Autodesk Inventor part; units mm, degrees
ref_plane "YZ Plane" through (0, 0, 0) normal (1, 0, 0) x (0, 1, 0)
ref_plane "XZ Plane" through (0, 0, 0) normal (0, 1, 0) x (-1, 0, 0)
ref_plane "XY Plane" through (0, 0, 0) normal (0, 0, 1) x (1, 0, 0)
sketch "Sketch1" plane through (0, 0, 0) normal (0, 0, 1) x (1, 0, 0)
  circle A0 centre (0, 0) radius 12.7
  circle A1 centre (0, 0) radius 50.8
  line L0 (50.8, 0) -> (50.8, -225.3234)
  line L1 (50.8, -225.3234) -> (-50.8, -225.3234)
  line L2 (-50.8, -225.3234) -> (-50.8, 0)
  line L3 (-50.8, 0) -> (-12.7, 0)
  line L4 (12.7, 0) -> (50.8, 0)
  dimension "d1" = 101.6
  dimension "d0" = 25.4
  dimension "d2" = 225.3234
extrude "Extrusion1" add sketch "Sketch1" along normal blind 12.7 contours L4 A1 L3 A0 | A0 L3 A1 L4 | L0 L1 L2 A1
sketch "Sketch2" plane through (0, 0, 12.7) normal (0, 0, 1) x (1, 0, 0)
  circle A0 centre (0, 0) radius 12.7
  arc A1 (50.8, 0) -> (-50.8, 0) centre (0, 0) ccw
  line L0 (-50.8, 0) -> (-50.8, -225.3234)
  line L1 (-50.8, -225.3234) -> (50.8, -225.3234)
  line L2 (50.8, -225.3234) -> (50.8, 0)
  circle A2 centre (176.5046, -179.1208) radius 32.385
  circle A3 centre (253.9746, -179.1208) radius 32.385
  line L3 (144.1196, -225.3234) -> (144.1196, -179.1208)
  line L4 (286.3596, -225.3234) -> (286.3596, -179.1208)
  line L5 (176.5046, -146.7358) -> (253.9746, -146.7358)
  line L6 (50.8, -225.3234) -> (144.1196, -225.3234)
  line L7 (286.3596, -225.3234) -> (508, -225.3234)
  line L8 (-50.8, -225.3234) -> (-238.2266, -225.3234)
  line L9 (-263.6266, -225.3234) -> (-263.6266, -150.876)
  line L10 (-263.6266, -150.876) -> (-212.8266, -150.876)
  line L11 (-212.8266, -150.876) -> (-212.8266, 50.8)
  line L12 (-212.8266, 50.8) -> (508, 50.8)
  line L13 (508, 50.8) -> (508, -225.3234)
  line L14 (-238.2266, -229.108) -> (-238.2266, -225.3234)
  line L15 (-238.2266, -229.108) -> (-263.6266, -229.108)
  line L16 (-263.6266, -229.108) -> (-263.6266, -225.3234)
  dimension "d5" = 176.5046
  dimension "d6" = 179.1208
  dimension "d7" = 64.77
  dimension "d8" = 64.77
  dimension "d9" = 77.47
  dimension "d11" = 212.8266
  dimension "d13" = 50.8
  dimension "d16" = 150.876
  dimension "d17" = 508
  dimension "d18" = 229.108
extrude "Extrusion2" add sketch "Sketch2" against normal blind 12.7 contours A1 L12 L13 L7 L4 A3 L5 A2 L3 L6 L2 | A1 L0 L8 L14 L15 L16 L9 L10 L11 L12
sketch "Sketch3" plane through (0, 0, 12.7) normal (0, 0, 1) x (1, 0, 0)
  circle A0 centre (0, 0) radius 12.7
  circle A1 centre (225.0958, -205.5114) radius 12.7
  dimension "d19" = 25.4
  dimension "d20" = 304.8
  dimension "d21" = 205.5114
sketch "Sketch4" plane through (0, 0, 12.7) normal (0, 0, 1) x (1, 0, 0)
  line L0 (144.1196, -225.3234) -> (106.0196, -225.3234)
  line L1 (106.0196, -225.3234) -> (106.0196, -136.4234)
  line L2 (106.0196, -136.4234) -> (144.1196, -136.4234)
  line L3 (144.1196, -136.4234) -> (144.1196, -225.3234)
  line L4 (286.3596, -225.3234) -> (324.4596, -225.3234)
  line L5 (324.4596, -225.3234) -> (324.4596, -136.4234)
  line L6 (324.4596, -136.4234) -> (286.3596, -136.4234)
  line L7 (286.3596, -136.4234) -> (286.3596, -225.3234)
  dimension "d22" = 38.1
  dimension "d23" = 88.9
  dimension "d24" = 38.1
  dimension "d25" = 88.9
extrude "Extrusion3" add sketch "Sketch4" along normal blind 25.4
sketch "Sketch5" plane through (0, 0, 38.1) normal (0, 0, 1) x (1, 0, 0)
  line L0 (106.0196, -136.4234) -> (324.4596, -136.4234)
  line L1 (324.4596, -136.4234) -> (324.4596, -225.3234)
  line L2 (324.4596, -225.3234) -> (106.0196, -225.3234)
  line L3 (106.0196, -225.3234) -> (106.0196, -136.4234)
  point P0 (0, 0)
  dimension "d28" = 218.44
extrude "Extrusion4" add sketch "Sketch5" along normal blind 12.7
extrude "Extrusion5" cut sketch "Sketch3" along normal blind 76.2 contours A1
sketch "Sketch6" plane through (0, 0, 12.7) normal (0, 0, 1) x (1, 0, 0)
  line L0 (324.4596, -136.4234) -> (324.4596, -225.3234)
  line L1 (324.4596, -225.3234) -> (508, -225.3234)
  line L2 (508, -225.3234) -> (508, 50.8)
  line L3 (324.4596, -136.4234) -> (508, -22.1234)
  dimension "d33" = 203.2
extrude "Extrusion6" cut sketch "Sketch6" against normal blind 25.4
sketch "Sketch7" plane through (0, 0, 50.8) normal (0, 0, 1) x (1, 0, 0)
  line L0 (106.0196, -136.4234) -> (106.0196, -225.3234)
  line L1 (324.4596, -225.3234) -> (324.4596, -136.4234)
  line L2 (324.4596, -136.4234) -> (106.0196, -136.4234)
  arc A0 (324.4596, -225.3234) -> (235.5596, -136.4234) centre (235.5596, -225.3234) ccw
  line L3 (324.4596, -225.3234) -> (235.5596, -136.4234) construction
  line L4 (324.4596, -225.3234) -> (450.1832, -225.3234) construction
  arc A1 (194.9196, -136.4234) -> (106.0196, -225.3234) centre (194.9196, -225.3234) ccw
  line L5 (106.0196, -225.3234) -> (194.9196, -136.4234) construction
  line L6 (106.0196, -225.3234) -> (231.7432, -225.3234) construction
  point P0 (0, 0)
  dimension "d36" = 135
  dimension "d37" = 45
extrude "Extrusion7" cut sketch "Sketch7" against normal blind 38.1
fillet "Fillet1" radius 12.7 3 edges at (215.2396, -136.4234, 50.8) (298.4214, -162.4616, 50.8) (132.0578, -162.4616, 50.8)
sketch "Sketch8" plane through (0, 0, 0) normal (0, 0, -1) x (-1, 0, 0)
  line L0 (-508, 50.8) -> (-508, -22.1234)
  circle A0 centre (0, 0) radius 12.7
  line L1 (0, 0) -> (-271.2669, 0)
  circle A1 centre (-271.2669, 0) radius 35.56
  dimension "d41" = 71.12
extrude "Extrusion8" cut sketch "Sketch8" against normal blind 25.4 contours A1
sketch "Sketch9" plane through (0, 0, 0) normal (0, 0, -1) x (-1, 0, 0)
  circle A0 centre (-271.2669, 0) radius 35.56
  line L0 (-324.4596, -136.4234) -> (-324.4596, -225.3234)
  line L1 (-324.4596, -225.3234) -> (-286.3596, -225.3234)
  line L2 (-286.3596, -225.3234) -> (-286.3596, -179.1208)
  arc A1 (-253.9746, -146.7358) -> (-286.3596, -179.1208) centre (-253.9746, -179.1208) ccw
  line L3 (-253.9746, -146.7358) -> (-176.5046, -146.7358)
  arc A2 (-144.1196, -179.1208) -> (-176.5046, -146.7358) centre (-176.5046, -179.1208) ccw
  line L4 (-144.1196, -179.1208) -> (-144.1196, -225.3234)
  line L5 (-144.1196, -225.3234) -> (238.2266, -225.3234)
  line L6 (238.2266, -225.3234) -> (238.2266, -229.108)
  line L7 (238.2266, -229.108) -> (263.6266, -229.108)
  line L8 (263.6266, -229.108) -> (263.6266, -150.876)
  line L9 (263.6266, -150.876) -> (212.8266, -150.876)
  line L10 (212.8266, -150.876) -> (212.8266, 50.8)
  line L11 (212.8266, 50.8) -> (-508, 50.8)
  line L12 (-508, 50.8) -> (-508, -22.1234)
  line L13 (-508, -22.1234) -> (-324.4596, -136.4234)
  circle A3 centre (0, 0) radius 12.7
properties part number "Shooter_TopMotorSupport"
Input: part model. Units: mm. Frame: model coordinates. A direction names the side the tool comes from. Give positions to 0.01 mm unless a question says otherwise; leave off trailing zeros. Order: outer loops, then holes, each group sorted by start corner. A loop starts at its lowest first (then second) coordinate and runs counter-clockwise, first axis right, second up.
1. Section C-C on z = 22. Return the cut outline in (x, y).
Derived:
outline: (106.02, -225.32) - (144.12, -225.32) - (144.12, -152.37) arc R88.9 ccw to start; (286.36, -225.32) - (324.46, -225.32) arc R88.9 ccw to (286.36, -152.37) - close
2. Section A-A on y = 0. Return the cut outline in (x, z), and give its area (3 significant figures).
Derived:
outline: (-212.83, 0) - (-12.7, 0) - (-12.7, 12.7) - (-212.83, 12.7) - close; (12.7, 0) - (235.71, 0) - (235.71, 12.7) - (12.7, 12.7) - close; (306.83, 0) - (508, 0) - (508, 12.7) - (306.83, 12.7) - close
area: 7,930 mm2
3. Pin query (flat end, axial travel): pin 1 (4 mm diameter, centred on x = 141, z = 26.5, fed in from +Y); pin 2 (1 mm diameter, centred on x = 342, z = 7.5, fed in from -Y); pin 3 (5 mm diameter, centred on x = 313, z = 35.5, fed in from -Y). Return the tip coordinate at first contact, or that it passes through.
Derived:
pin 1: stops at y = -153.16
pin 2: stops at y = -125.81
pin 3: stops at y = -225.32
4. Material intervals for L1, parallel to X at y = -177, z = 10; L2, parallel to Y at x = 308, z = 2; L3, parallel to Y at x = 233, z = 8, sorted ascending.
Derived:
L1: x = -263.63 to 144.19, 286.29 to 324.46
L2: y = -225.32 to 50.8
L3: y = -146.74 to 50.8
5. Mould query, pull axis Z, two halves, no side actions, for faces 4 (the flat face through (144.12, -189, 19)), 5 (the cylindrical face through (215.524, -140.045, 46.981)), 6 (the flat face through (-239, -150.876, 6)). Classes: released by +Z, released by -Z, zero draft, split by the parting line, or undercut.
Derived:
face 4: undercut
face 5: released by +Z
face 6: zero draft
6. Section D-D on x = 416. Return the cut outline in (y, z).
Derived:
outline: (-79.42, 0) - (50.8, 0) - (50.8, 12.7) - (-79.42, 12.7) - close
7. Section B-B on x = 0. Return the cut outline in (y, z).
Derived:
outline: (-225.32, 0) - (-12.7, 0) - (-12.7, 12.7) - (-225.32, 12.7) - close; (12.7, 0) - (50.8, 0) - (50.8, 12.7) - (12.7, 12.7) - close
8. Reachability of faces 1 (the flat face through (-212.827, -51, 6)), 2 (the cylindrical face through (153.86, -155.97, 6.44)), 3 (the flat face through (110, -225.323, 19)) from +Z, -Z, +X, -X, +Y, -Y: full face, straight path, thin tool, end or side. Return the list, or none.
Derived:
face 1: +Z, -Z, -X, +Y
face 2: -Z, -Y
face 3: +Z, -Z, +X, -Y
